The model under review builds one solid part; all positions refer to its coordinate system, in mm. Round coordinates to 2 decimals unless told otherwise and drop trailing zeros. Loops run counter-clockwise (first coordinate to the right, second up) from the corner with the lowest first, then second, coordinate; pieces in that order, holes last. Notation, with made-up numbers: M 83.5,55.25 L 100.5,55.25 A32 cw 100.5,90.25 Z; hole C -13.75,70 d2. An arc over 180 degrees is marked long. Return JSON: item names as keys, results as strings. Group by question number.
Q1. Clearance check with flat-ended pins moving along their axes: pin 1 Ø3 at (y, z) = (14.5, -2.5) entering from +X; pin 2 Ø1 at (x, y) = (-2.5, 14) entering from +Z; pin 3 Ø3 at (x, z) = (4, 2.5) entering from -Y. State where each tip first meets the part, or that it passes through.
Q2. Consider section C-C (x = -3.25). State the section outline as (y, z) points.
Q3. Consider section B-B (z = 2.5). State the section outline as (x, y) points.
Q4. Consider section A-A (y = 3.75). State the section outline as (x, z) points.
Q5. To check wall thickness, follow line 1 along X through (y, z) = (14.5, -3); line 2 along X through (y, z) = (3, -2.25); line 3 along Z through (x, y) = (3.75, 1). State the ranges of each line that lie inside material, in increasing order.
from build123d import *

# Parameters (mm, degrees)
EXTRUDE1_DEPTH = 20


with BuildPart() as part:
    # Sketch1 → Extrude1 (new body)
    with BuildSketch(Plane(origin=(0, 0, 0), x_dir=(1, 0, 0), z_dir=(0, 1, 0))):
        Polygon((4.253254042, -3.090169944), (5.257311121, 0), (4.253254042, 3.090169944), (1.624598481, 5), (-1.624598481, 5), (-4.253254042, 3.090169944), (-5.257311121, 0), (-4.253254042, -3.090169944), (-1.624598481, -5), (1.624598481, -5), align=None)
    extrude(amount=EXTRUDE1_DEPTH)


solid = part.part
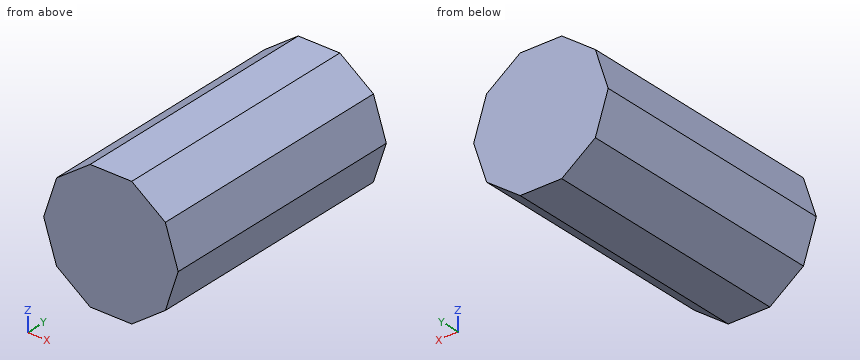
Values:
{
 "1": {"pin 1": "stops at x = 4.93", "pin 2": "stops at z = 4.73", "pin 3": "stops at y = 0"},
 "2": {"outline": "M 0,-3.82 L 20,-3.82 L 20,3.82 L 0,3.82 Z"},
 "3": {"outline": "M -4.45,0 L 4.45,0 L 4.45,20 L -4.45,20 Z"},
 "4": {"outline": "M -5.26,0 L -4.25,-3.09 L -1.62,-5 L 1.62,-5 L 4.25,-3.09 L 5.26,0 L 4.25,3.09 L 1.62,5 L -1.62,5 L -4.25,3.09 Z"},
 "5": {"line 1": "x = -4.28 to 4.28", "line 2": "x = -4.53 to 4.53", "line 3": "z = -3.46 to 3.46"}
}
